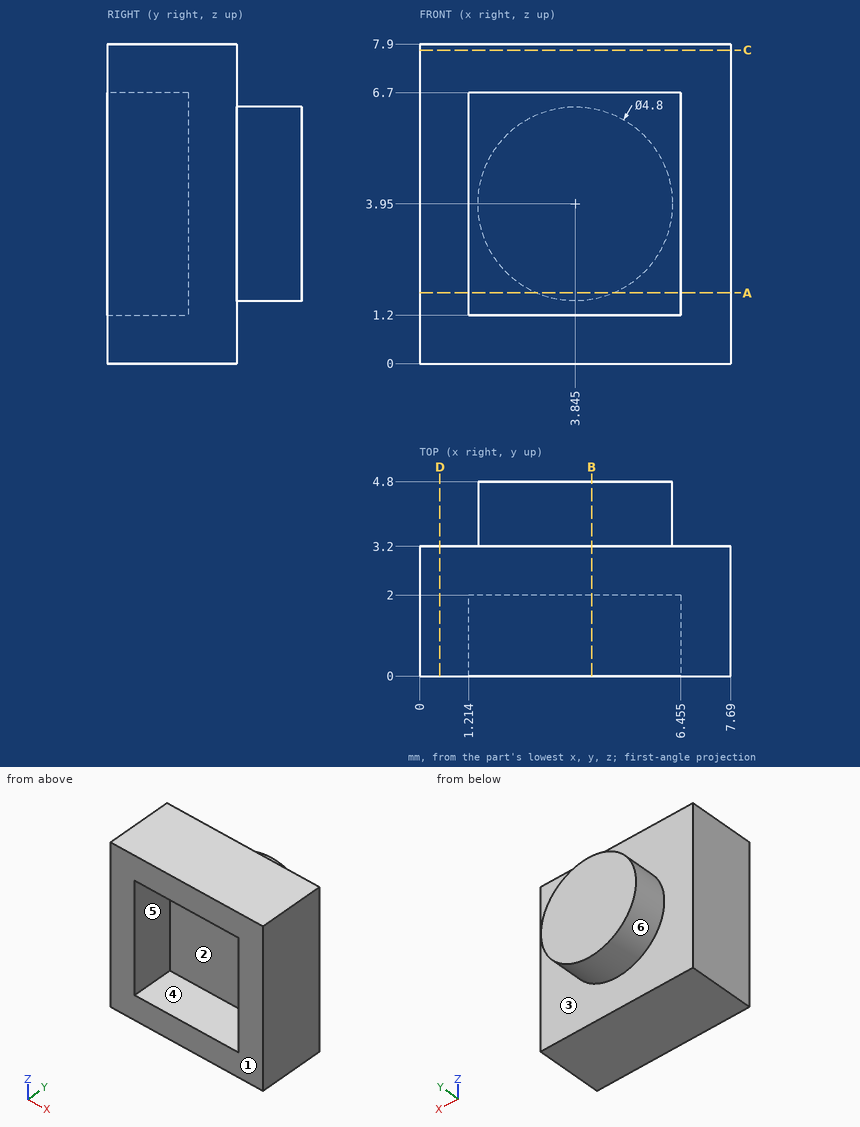
The figure shows three views and two pictorial views of one solid part (mm, origin at its lowest corner). Answer the questions. A direction names the side the tool comes from. Coordinates: 2 decimals unless noted, no trailing zeros. Write each loop counter-clockwise with the first axis right and the second up, starting at its lowest first coordinate (ties: lowest second). Pieces come first, ordered by that corner, then holes. Notation, with made-up numbers: (42, 24.25) -> (53, 24.25) arc R18 cw to (53, 35.25) -> close; hole circle Ø2 at (72, 48.5). An arc over 180 degrees is marked (long way). Answer as a JSON object with one key per item and string values.
Q1. The part is cut by section D-D on x = 0.5. Give the vertices of the cut face in (y, z).
The answers:
{"outline": "(0, 0) -> (3.2, 0) -> (3.2, 7.9) -> (0, 7.9) -> close"}
Q2. Determine the mould class of the marked faces 3, 4, 5 and 6 for opening direction Z: pulls with the +Z half, pulls with the -Z half, needs draft (parallel to the pull), parting line crosses it, or undercut.
The answers:
{"face 3": "needs draft", "face 4": "undercut", "face 5": "undercut", "face 6": "parting line crosses it"}
Q3. The part is cut by section C-C on z = 7.75. Give the vertices of the cut face in (x, y), then the cut area to 3 significant figures.
The answers:
{"outline": "(0, 0) -> (7.69, 0) -> (7.69, 3.2) -> (0, 3.2) -> close", "area": "24.6 mm2"}
Q4. The part is cut by section B-B on x = 4.25. Give the vertices of the cut face in (y, z), then the cut area to 4 significant figures.
The answers:
{"outline": "(0, 0) -> (3.2, 0) -> (3.2, 1.58) -> (4.8, 1.58) -> (4.8, 6.32) -> (3.2, 6.32) -> (3.2, 7.9) -> (0, 7.9) -> (0, 6.7) -> (2, 6.7) -> (2, 1.2) -> (0, 1.2) -> close", "area": "21.85 mm2"}
Q5. The part is cut by section A-A on z = 1.75. Give the vertices of the cut face in (x, y) (3 decimals).
The answers:
{"outline": "(0, 0) -> (1.214, 0) -> (1.214, 2) -> (6.455, 2) -> (6.455, 0) -> (7.69, 0) -> (7.69, 3.2) -> (4.804, 3.2) -> (4.804, 4.8) -> (2.886, 4.8) -> (2.886, 3.2) -> (0, 3.2) -> close"}
Q6. A tool of negligible diameter and unlimited length cuts with its end or side. For the marked faces 1 and 2, from which of +Z, -Z, +X, -X, +Y, -Y can it reach the whole face along a straight path? Write none if from no direction.
The answers:
{"face 1": "+Z, -Z, +X, -X, -Y", "face 2": "-Y"}
Q7. Consider line 1 (X direction, y = 0.75, z = 4) (3 decimals); line 2 (Z direction, x = 3.5, y = 1.2); line 3 (Y direction, x = 0.5, z = 5.5). Determine where each line is inside the solid, lowest interval first. Write a range as [from, to].
The answers:
{"line 1": "x = [0, 1.214], [6.455, 7.69]", "line 2": "z = [0, 1.2], [6.7, 7.9]", "line 3": "y = [0, 3.2]"}
